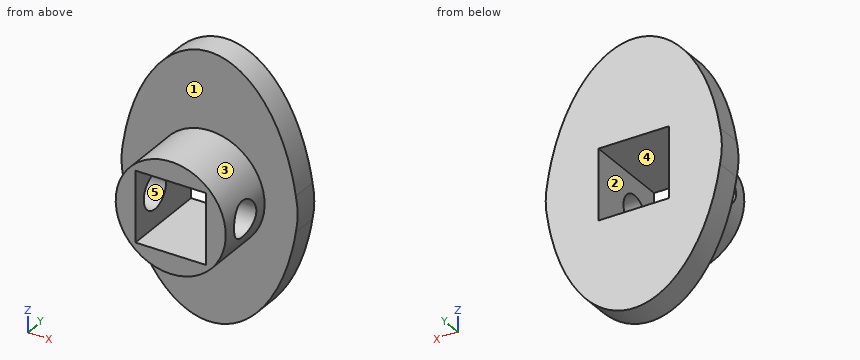
from build123d import *

# Parameters (mm, degrees)
BOSS_EXTRUDE1_DEPTH     = 3.81
SKETCH3_R               = 7.9375
BOSS_EXTRUDE2_DEPTH     = 8.89
SKETCH2_W               = 10.16
SKETCH2_H               = 10.16
CUT_EXTRUDE1_DEPTH      = 27.181720844
CUT_EXTRUDE2_DEPTH      = 30.459141437
CUT_EXTRUDE2_DEPTH_BACK = 30.459141437
SKETCH4_R               = 2.55


# Read off the part's stored shape, not the designer's step: Boss-Extrude1
with BuildPart() as part:
    # Boss-Extrude1 outline → Boss-Extrude1 (new body)
    with BuildSketch(Plane(origin=(0, 0, 0), x_dir=(1, 0, 0), z_dir=(0, 1, 0))):
        with BuildLine():
            ThreePointArc((12.443407893, -2.54), (12.7, 0), (12.443407893, 2.54))
            add(Edge.make_bspline(
                [(-12.443407893, 2.54), (0, 83.206957613), (12.443407893, 2.54)],
                knots=[0, 0, 0, 1, 1, 1], degree=2, weights=[1, 0.257337639, 1]))
            ThreePointArc((-12.443407893, 2.54), (-12.7, 0), (-12.443407893, -2.54))
            add(Edge.make_bspline(
                [(-12.443407893, -2.54), (0, -83.206957613), (12.443407893, -2.54)],
                knots=[0, 0, 0, 1, 1, 1], degree=2, weights=[1, 0.257337639, 1]))
        make_face()
    extrude(amount=BOSS_EXTRUDE1_DEPTH)

    # Sketch3 → Boss-Extrude2 (add)
    with BuildSketch(Plane.XZ):
        with Locations(Location((0, 0, 0), (0, 0, 270))):
            Circle(SKETCH3_R)
    extrude(amount=BOSS_EXTRUDE2_DEPTH)

    # Sketch2 → Cut-Extrude1 (cut, through all)
    with BuildSketch(Plane(origin=(0, 3.81, 0), x_dir=(1, 0, 0), z_dir=(0, 1, 0))):
        Rectangle(SKETCH2_W, SKETCH2_H)
    extrude(amount=-CUT_EXTRUDE1_DEPTH, mode=Mode.SUBTRACT)

    # Sketch4 → Cut-Extrude2 (cut, two sides: drawn at the far end of the back side and taken through both)
    with BuildSketch(Plane(origin=(7.9375, 0, 0), x_dir=(0, 0, -1), z_dir=(1, 0, 0)).offset(-CUT_EXTRUDE2_DEPTH_BACK)):
        with Locations((0, -4.445)):
            Circle(SKETCH4_R)
    extrude(amount=CUT_EXTRUDE2_DEPTH + CUT_EXTRUDE2_DEPTH_BACK, mode=Mode.SUBTRACT)


solid = part.part
Check sheet for the modelled part. Datum: model origin and axes. Units: mm. Face numbers are marked on the shaded views. A direction names the side the tool comes from. Coordinates: 2 decimals unless noted, no trailing zeros. Write each loop counter-clockwise with the first axis right and the second up, starting at its lowest first coordinate (ties: lowest second). Pieces come first, ordered by that corner, then holes. Notation, with made-up numbers: M -32,52 L -7,52 A20 cw -7,86 Z; hole C -36.5,66 d7. An arc over 180 degrees is marked long. Answer as CSV lines item,"result".
Q1. Cross-section at A-A (z = 0). Record the boundary of the cut face in (x, y) (1 decimal), then the cut area to 3 significant figures.
Check result:
outline,"M -12.7,0 L -7.9,0 L -7.9,-1.9 L -5.1,-1.9 L -5.1,3.8 L -12.7,3.8 Z; M -7.9,-8.9 L -5.1,-8.9 L -5.1,-7 L -7.9,-7 Z; M 5.1,-8.9 L 7.9,-8.9 L 7.9,-7 L 5.1,-7 Z; M 5.1,-1.9 L 7.9,-1.9 L 7.9,0 L 12.7,0 L 12.7,3.8 L 5.1,3.8 Z"
area,"79.7 mm^2"
Q2. Go/stop test with flat-tipped pins: pin 1 (4 mm diameter, centred on y = -4.445, z = 0, fed in from +X); pin 2 (2 mm diameter, centred on y = 1.5, z = 4, fed in from +X); pin 3 (3 mm diameter, centred on y = -1, z = 2, fed in from -X); pin 4 (3 mm diameter, centred on x = 7, y = -4.5, fed in from +Z). Record where each tip stops, or that it passes through.
Check result:
pin 1,"through"
pin 2,"x = 12.37"
pin 3,"x = -12.67"
pin 4,"z = 5.72"
Q3. Cross-section at C-C (y = -5.25). Record the boundary of the cut face in (x, z) (1 decimal), then the cut area to 3 significant figures.
Check result:
outline,"M -7.6,-2.4 A7.9 ccw 7.6,-2.4 L 5.1,-2.4 L 5.1,-5.1 L -5.1,-5.1 L -5.1,-2.4 Z; M -7.6,2.4 L -5.1,2.4 L -5.1,5.1 L 5.1,5.1 L 5.1,2.4 L 7.6,2.4 A7.9 ccw Z"
area,"68.3 mm^2"
Q4. Material ranges on probe 1 along Y at (x, z) = (7.35, 0) (3 decimals); probe 2 along Z at (x, y) = (0, 1); probe 3 along Y at (x, z) = (-9.75, -8.5), recorded low to high. Write a range as from..to.
Check result:
probe 1,"-8.89..-6.995, -1.895..3.81"
probe 2,"-19.05..-5.08, 5.08..19.05"
probe 3,"0..3.81"
Q5. Cross-section at B-B (y = -1.25). Record the boundary of the cut face in (x, z) (1 decimal).
Check result:
outline,"C 0,0 d15.9; hole M -5.1,-5.1 L 5.1,-5.1 L 5.1,5.1 L -5.1,5.1 Z"
Q6. Set-up check for the marked faces 4 and 5: record each of +Z, -Z, +X, -X, +Y, -Y from which the full face is reachable in a straight line by a thin tool's end or side.
Check result:
face 4,"+Y, -Y"
face 5,"+X, -X"
Q7. Mould release check, pull along X, two halves, no side actions. Record for the marked faces 1, 2 and 3: released by +X, released by -X, zero draft, split by the parting line, or undercut.
Check result:
face 1,"zero draft"
face 2,"undercut"
face 3,"split by the parting line"
